Part model, mm, in its own coordinate system. Round coordinates to 2 decimals unless told otherwise and drop trailing zeros. Write each loop counter-clockwise with the first axis right and the second up, starting at its lowest first coordinate (ties: lowest second). Pieces come first, ordered by that corner, then holes. Notation, with made-up numbers: (62.25, 79) -> (86.25, 79) arc R17 cw to (86.25, 90) -> close; hole circle Ø4 at (-9, 64). An arc over 180 degrees is marked (long way). Return JSON: item names as keys, results as strings. Group by question number.
(1) Mould opens along Z. For faces 1 (the cylindrical face through (50.731, 1.208, 92.492)), 2 (the flat face through (52, 1, 10)), 3 (the flat face through (32, 0, 62)) say: +Z half, -Z half, draft (parallel to the pull), parting line (faces both ways), or undercut.
(2) Saw through at A-A (y = 0.5). List the corners of the cut face in (x, z).
(3) Drop a flat-ended pin along its axis: pin 1 Ø2.5 at (x, z) = (2.5, 86) entering from -Y. Give the stop position or say it passes through.
(4) Drill centre lines: L1, parallel to X at y = 1.3, z = 21; L2, parallel to Z at x = 2.5, y = 0.45; L3, parallel to Z at x = 50.5, y = 1.3. Where is each one in solid material? Low to high. Write a range as from..to.
Autodesk Inventor part; units mm, degrees
ref_plane "YZ Plane" through (0, 0, 0) normal (1, 0, 0) x (0, 1, 0)
ref_plane "XZ Plane" through (0, 0, 0) normal (0, 1, 0) x (-1, 0, 0)
ref_plane "XY Plane" through (0, 0, 0) normal (0, 0, 1) x (1, 0, 0)
sketch "Skizze1" plane through (0, 0, 0) normal (0, 1, 0) x (-1, 0, 0)
  line L0 (0, 0) -> (-42, 0)
  line L1 (-63, 21) -> (-63, 123)
  line L2 (-63, 123) -> (0, 123)
  line L3 (0, 123) -> (0, 0)
  line L4 (-42, 0) -> (-63, 21)
  line L5 (-42, 0) -> (-12.3015, 0) construction
  circle A0 centre (-14, 5) radius 3.5
  circle A1 centre (-32, 21) radius 1.5
  circle A2 centre (-2.5, 86) radius 1.5
  circle A3 centre (-50.5, 89) radius 3.5
  dimension "d0" = 63
  dimension "d1" = 102
  dimension "d2" = 135
  dimension "d3" = 42
  dimension "d4" = 7
  dimension "d5" = 3
  dimension "d6" = 3
  dimension "d7" = 7
  dimension "d8" = 2.5
  dimension "d9" = 37
  dimension "d10" = 14
  dimension "d11" = 5
  dimension "d12" = 21
  dimension "d13" = 32
  dimension "d14" = 12.5
  dimension "d15" = 34
extrude "Extrusion1" add sketch "Skizze1" along normal blind 1
sketch "Sketch2" plane through (0, 1, 0) normal (0, 1, 0) x (1, 0, 0)
  circle A0 centre (50.5, -89) radius 3.5
  circle A1 centre (14, -5) radius 3.5
  circle A2 centre (2.5, -86) radius 1.5
  circle A3 centre (32, -21) radius 1.5
  line L0 (42, 0) -> (0, 0)
  line L1 (0, 0) -> (0, -123)
  line L2 (0, -123) -> (63, -123)
  line L3 (63, -123) -> (63, -21)
  line L4 (63, -21) -> (42, 0)
extrude "Extrusion2" add sketch "Sketch2" along normal blind 1
properties part number "01_PCBoard"
Computed values:
{
 "1": {"face 1": "undercut", "face 2": "-Z half", "face 3": "draft"},
 "2": {"outline": "(0, 0) -> (42, 0) -> (63, 21) -> (63, 123) -> (0, 123) -> close; hole circle Ø3 at (2.5, 86); hole circle Ø7 at (14, 5); hole circle Ø3 at (32, 21); hole circle Ø7 at (50.5, 89)"},
 "3": {"pin 1": "through"},
 "4": {"L1": "0..30.5, 33.5..63", "L2": "0..84.5, 87.5..123", "L3": "8.5..85.5, 92.5..123"}
}
